The listing builds one solid part. Answer for the finished solid, in the listing's coordinates (mm). A direction names the side the tool comes from. Give positions to 0.01 mm unless a question says otherwise; leave off trailing zeros. Write each loop counter-clockwise with the first axis right and the second up, starting at its lowest first coordinate (ties: lowest second). Pieces come first, ordered by that corner, then holes. Notation, with made-up numbers: (-1.75, 63.25) -> (35.25, 63.25) arc R12 cw to (35.25, 80.25) -> close; hole circle Ø9 at (70.25, 79). An arc over 180 degrees is marked (long way). Use CSV: the item, a comma, the result in double quotes. Start each with the question number.
from build123d import *

# Parameters (mm, degrees)
F1_DEPTH  = 20
F2_R      = 2.5
F3_T      = -1.6
F4_R      = 4.05
F4_R_2    = 2.25
F5_DEPTH  = 20
F6_W      = 18.5
F6_H      = 6.8
F7_DEPTH  = 7.7
F9_R      = 11.6656058432
F10_DEPTH = 24.5
F11_R     = 3.5
F12_R     = 1
F4_R_3    = 2.65
F13_DEPTH = 25


with BuildPart() as f1:
    # F0 (on Top) → F1 (new body)
    with BuildSketch(Plane.XY):
        with BuildLine():
            ThreePointArc((-65, 0), (-45.9619407771, 45.9619407771), (0, 65))
            Line((0, 65), (-65, 65))
            Line((-65, 65), (-65, 60))
            Line((-65, 60), (-65, 41.2))
            Line((-65, 41.2), (-65, 0))
        make_face()
    extrude(amount=F1_DEPTH)

    # F2
    f2_edges = [f1.edges().sort_by_distance(p)[0] for p in [
        (-65, 0, 10),
        (0, 65, 10),
        (-65, 65, 10),
    ]]
    fillet(f2_edges, radius=F2_R)

    # F3
    f3_openings = [f1.faces().sort_by_distance(p)[0] for p in [
        (-51.245763, 51.245763, 0),
    ]]
    offset(amount=F3_T, openings=f3_openings)

    # F4 (on face) → F5 (join)
    with BuildSketch(Plane.XY.offset(20)):
        with Locations((-60.9282360965, 60.9400444936)):
            Circle(F4_R)
        with Locations((-60.9282360965, 60.9400444936)):
            Circle(F4_R_2, mode=Mode.SUBTRACT)
        with Locations((-60.8160617149, 34.0815317436)):
            Circle(F4_R)
        with Locations((-60.8160617149, 34.0815317436)):
            Circle(F4_R_2, mode=Mode.SUBTRACT)
        with Locations((-34.0815317436, 60.8160617149)):
            Circle(F4_R)
        with Locations((-34.0815317436, 60.8160617149)):
            Circle(F4_R_2, mode=Mode.SUBTRACT)
    extrude(amount=-F5_DEPTH)

    # F6 (on face) → F7 (cut)
    with BuildSketch(Plane(origin=(-65, 0, 0), x_dir=(0, -1, 0), z_dir=(-1, 0, 0))):
        with Locations((-47.55, 3.4)):
            Rectangle(F6_W, F6_H)
    extrude(amount=-F7_DEPTH, mode=Mode.SUBTRACT)

    # F9 (on face) → F10 (cut)
    with BuildSketch(Plane(origin=(-32.5, 32.5, 0), x_dir=(-0.7071067812, -0.7071067812, 0), z_dir=(-0.7071067812, 0.7071067812, 0))):
        with Locations((0.8223271579, 0)):
            Circle(F9_R)
    extrude(amount=F10_DEPTH, mode=Mode.SUBTRACT)

    # F11
    f11_edges = [f1.edges().sort_by_distance(p)[0] for p in [
        (-64.2, 38.3, 6.8),
        (-64.2, 56.8, 6.8),
    ]]
    fillet(f11_edges, radius=F11_R)

    # F12
    f12_edges = [f1.edges().sort_by_distance(p)[0] for p in [
        (-45.961941, 45.961941, 20),
        (-23.041831, 62.981125, 20),
        (-43.997549, 65, 20),
        (-62.981125, 23.041831, 20),
        (-65, 43.997549, 20),
    ]]
    fillet(f12_edges, radius=F12_R)

    # F4 (on face) → F13 (cut)
    with BuildSketch(Plane.XY.offset(20)):
        with Locations((-58.35, 52.85)):
            Circle(F4_R_3)
        with Locations((-46.35, 52.85)):
            Circle(F4_R_3)
    extrude(amount=-F13_DEPTH, mode=Mode.SUBTRACT)


solid = f1.part
Q1. Section A-A on z = 1.5 is taken. State how many separate pieces and enclosed holes the cut face has, then the cut area to 3 significant figures.
Q2. Flat-ended cylindrical pins translate along their axes: pin 1 Ø5 at (y, z) = (46, 13.5) entering from +X; pin 2 Ø4.5 at (x, y) = (-61, 27.5) entering from -Z; pin 3 Ø0.5 at (x, z) = (-64.5, 2.5) entering from +Y; pin 4 Ø1 at (x, z) = (-53, 6.5) entering from -Y. Find the tip coordinate at first contact, or state that the pin passes through.
Q3. Section B-B on z = 13 is taken. Give the vertices of the cut face in (x, y).
Q4. The mould has two halves that part along Y. Classify faces 4 (the face through (-23.033, 62.934, 9.633)), 5 (the face through (-44, 65, 9)), 6 (the face through (-63.4, 48, 11)), 7 (the face through (-61, 31, 0)): +Y half, -Y half, draft (parallel to the pull), parting line (faces both ways), or undercut.
Q5. For faces 1 (the face through (-64, 56.8, 2)), 2 (the face through (-24.61, 62.66, 9.33)), 3 (the face through (-64.19, 39.3, 5.75)), determine the directions among +Z, -Z, +X, -X, +Y, -Y from which every point of the face is accessible in a straight line to the end or side of a thin tool.
Q6. Straight lines are drawn through the part: L1, parallel to Y at x = -60, z = 4.5; L2, parallel to Y at x = -41, z = 1.25; L3, parallel to Y at x = -59, z = 4.5. For each, find the intervals that lie inside material, in ascending order.
Output:
1,separate pieces,"2"
1,enclosed holes,"5"
1,area,"228 mm²"
2,pin 1,"x = -43.28"
2,pin 2,"z = 0"
2,pin 3,"y = 64.29"
2,pin 4,"y = 36.92"
3,outline,"(-65, 25.5) arc R2.5 ccw to (-60.19, 24.55) arc R65 cw to (-24.55, 60.19) arc R2.5 ccw to (-25.5, 65) -> (-62.5, 65) arc R2.5 ccw to (-65, 62.5) -> close; hole (-63.4, 25.5) arc R0.9 ccw to (-61.67, 25.16) arc R66.6 cw to (-59.29, 30.33) arc R4.05 cw to (-63.4, 30.96) -> close; hole (-63.4, 37.2) arc R4.05 cw to (-56.82, 34.74) arc R66.6 cw to (-34.74, 56.82) arc R4.05 cw to (-37.2, 63.4) -> (-57.71, 63.4) arc R4.05 cw to (-63.4, 57.73) -> close; hole circle Ø4.5 at (-60.93, 60.94); hole circle Ø4.5 at (-60.82, 34.08); hole circle Ø4.5 at (-34.08, 60.82); hole (-30.96, 63.4) arc R4.05 cw to (-30.33, 59.29) arc R66.6 cw to (-25.16, 61.67) arc R0.9 ccw to (-25.5, 63.4) -> close"
4,face 4,"parting line"
4,face 5,"+Y half"
4,face 6,"undercut"
4,face 7,"draft"
5,face 1,"-Z, -X"
5,face 2,"-Z"
5,face 3,"-Z, +X, -X"
6,L1,"25 to 28.91, 30.11 to 31.98, 36.18 to 38.05, 57 to 58.89, 62.99 to 65"
6,L2,"63.4 to 65"
6,L3,"27.28 to 32.75, 35.41 to 37.7, 57.38 to 59.78, 62.1 to 65"
